from build123d import *

# Parameters (mm, degrees)
SKETCH1_R           = 13
BOSS_EXTRUDE1_DEPTH = 32
SKETCH2_R           = 3.175
CUT_EXTRUDE1_DEPTH  = 37.905284174
SKETCH3_R           = 5
CUT_EXTRUDE2_DEPTH  = 20
CHAMFER1_SIZE       = 1


with BuildPart() as part:
    # Sketch1 → Boss-Extrude1 (new body)
    with BuildSketch(Plane(origin=(0, 0, 0), x_dir=(0, 0, -1), z_dir=(1, 0, 0))):
        Circle(SKETCH1_R)
    extrude(amount=BOSS_EXTRUDE1_DEPTH)

    # Sketch2 → Cut-Extrude1 (cut, through all)
    with BuildSketch(Plane(origin=(32, 0, 0), x_dir=(0, 0, -1), z_dir=(1, 0, 0))):
        Circle(SKETCH2_R)
    extrude(amount=-CUT_EXTRUDE1_DEPTH, mode=Mode.SUBTRACT)

    # Sketch3 → Cut-Extrude2 (cut)
    with BuildSketch(Plane.ZY):
        Circle(SKETCH3_R)
    extrude(amount=-CUT_EXTRUDE2_DEPTH, mode=Mode.SUBTRACT)

    # Chamfer1
    chamfer1_edges = [part.edges().sort_by_distance(p)[0] for p in [
        (0, 0, 13),
        (32, 0, 13),
    ]]
    chamfer(chamfer1_edges, length=CHAMFER1_SIZE)


solid = part.part
CAD build for the part. Positions are in the model's coordinates, mm. A direction names the side the tool comes from. Give positions to 0.01 mm unless a question says otherwise; leave off trailing zeros. Write each loop counter-clockwise with the first axis right and the second up, starting at its lowest first coordinate (ties: lowest second). Pieces come first, ordered by that corner, then holes. Notation, with made-up numbers: (16.5, 75.25) - (28.5, 75.25) arc R24 ccw to (28.5, 105.25) - close; hole circle Ø4 at (-16, 36). An arc over 180 degrees is marked (long way). Answer as CSV lines item,"result".
Q1. Band-saw the part on A-A (z = 0). Give the cut face in (x, y) (3 decimals), and give its area (3 significant figures).
Result set:
outline,"(0, -12) - (1, -13) - (31, -13) - (32, -12) - (32, -3.175) - (20, -3.175) - (20, -5) - (0, -5) - close; (0, 5) - (20, 5) - (20, 3.175) - (32, 3.175) - (32, 12) - (31, 13) - (1, 13) - (0, 12) - close"
area,"554 mm²"
Q2. Flat gauge pins, fed straight in: pin 1 Ø5 at (x, z) = (17, -5) entering from +Y; pin 2 Ø1.5 at (x, z) = (28.5, -10) entering from +Y; pin 3 Ø8 at (x, y) = (19, -5.5) entering from +Z. Where does each tip first touch, or does it go through?
Result set:
pin 1,"y = 12.76"
pin 2,"y = 9.13"
pin 3,"z = 12.91"
Q3. Drill centre lines: line 1 (Y direction, x = 4.5, z = 0); line 2 (Y direction, x = 28.25, z = 0) (3 decimals); line 3 (X direction, y = -0.25, z = -4.5). Where is each one in solid material? Low to high. Write a range as from..to.
Result set:
line 1,"-13..-5, 5..13"
line 2,"-13..-3.175, 3.175..13"
line 3,"20..32"
Q4. Band-saw the part on D-D (x = 26). Give the cut face in (y, z) (3 decimals), and give its area (3 significant figures).
Result set:
outline,"circle Ø26 at (0, 0); hole circle Ø6.35 at (0, 0)"
area,"499 mm²"
Q5. Band-saw the part on C-C (x = 9). Give the cut face in (y, z), and give its area (3 significant figures).
Result set:
outline,"circle Ø26 at (0, 0); hole circle Ø10 at (0, 0)"
area,"452 mm²"
Q6. Pull direction Y, two halves, no side cores. Call faces 3 (the face through (20, -3.3, 1)), 4 (the face through (15.79, -7.91, 10.316)), 5 (the face through (0, 0.2, -5.2)): released by +Y, released by -Y, zero draft, split by the parting line, or undercut.
Result set:
face 3,"undercut"
face 4,"split by the parting line"
face 5,"zero draft"
Q7. 3-axis set-ups, long thin cutter, end or side, ignore diameter. For faces 1 (the face through (9.86, -4.88, -1.08)), 2 (the face through (32, -2.5, -2.5)): which of +Z, -Z, +X, -X, +Y, -Y reach the whole face in a straight line?
Result set:
face 1,"-X"
face 2,"+Z, -Z, +X, +Y, -Y"
